Can you work these out from the model? Positions are in its coordinate system, mm. A direction names the side the tool comes from. Coordinates: 2 decimals unless noted, no trailing zeros. Order: outer loops, then holes, each group sorted by start corner. A loop starts at its lowest first (then second) coordinate and runs counter-clockwise, first axis right, second up. Notation, with made-up numbers: (73, 20.25) -> (81, 20.25) arc R28 ccw to (81, 39.25) -> close; hole circle Ø4 at (51.5, 17). An arc over 180 degrees is marked (long way). Answer as a JSON object with one key per item and string values. Group by question number.
(1) I want a section at C-C, the plane x = -25. List the corners of the cut face in (y, z) for me.
(2) For pin 1 (1.5 mm diameter, centred on x = -16.5, z = 11, fed in from -Y); pin 2 (1.3 mm diameter, centred on x = -11.5, z = -2.5, fed in from -Y); pin 3 (12 mm diameter, centred on y = -8.5, z = -16.5, fed in from +X); pin 4 (1.5 mm diameter, centred on y = -1.5, z = -11.5, fed in from -X), each with a flat end and sliding along its axis, tell me the tip position at first contact or that it passes through.
(3) I want a section at A-A, the plane y = 5.5. List the corners of the cut face in (x, z) for me, plus the area to 3 significant figures.
(4) Which directions (+Z, -Z, +X, -X, +Y, -Y) give clear straight access to the entire face, cutting with the end or side of a thin tool? Please do faces 4 (the flat face through (11, -5, 0)), 5 (the flat face through (-11, -5, 0)), 6 (the flat face through (0, -5, -11)), 7 (the flat face through (0, -5, 11)).
(5) I want a section at D-D, the plane y = -0.75. List the corners of the cut face in (x, z) for me, plus the area to 3 significant figures.
(6) I need wall thicknesses on line 1 (X direction, y = -9, z = 13.5); line 2 (Z direction, x = 23, y = -11.25); line 3 (Y direction, x = 12, z = 3). Which ranges of each line are inside material? Lowest first, please.
(7) If we mould it in two halves opening along Z, with no side actions, what happens to faces 1 (the cylindrical face through (21.166, -8.944, 21.26)), 2 (the cylindrical face through (8.64, 4.06, -9.08)), 3 (the flat face through (-15, -5, -15))? For each: pulls with the +Z half, pulls with the -Z half, needs draft (parallel to the pull), parting line crosses it, or undercut.
(8) I want a section at B-B, the plane z = -15. State how many separate pieces and enclosed holes the cut face has, plus the area to 3 significant figures.
Autodesk Inventor part; units mm, degrees
ref_plane "YZ Plane" through (0, 0, 0) normal (1, 0, 0) x (0, 1, 0)
ref_plane "XZ Plane" through (0, 0, 0) normal (0, 1, 0) x (-1, 0, 0)
ref_plane "XY Plane" through (0, 0, 0) normal (0, 0, 1) x (1, 0, 0)
sketch "スケッチ1" plane through (0, 0, 0) normal (0, 1, 0) x (-1, 0, 0)
  circle A0 centre (0, 0) radius 25
  circle A1 centre (0, 0) radius 30
  dimension "d0" = 50
  dimension "d1" = 60
extrude "押し出し1" add sketch "スケッチ1" along normal blind 8 contours A0 | A1
sketch "スケッチ2" plane through (0, 8, 0) normal (0, 1, 0) x (1, 0, 0)
  circle A0 centre (0, 0) radius 30
  line L0 (0, -30) -> (-30, 0)
  line L1 (-30, 0) -> (0, 30)
  line L2 (0, 30) -> (30, 0)
  line L3 (0, -30) -> (30, 0)
  circle A1 centre (0, 0) radius 30
  circle A2 centre (0, 0) radius 25
  circle A3 centre (-23, 23) radius 20
  circle A4 centre (-23, -23) radius 20
  circle A5 centre (23, -23) radius 20
  circle A6 centre (23, 23) radius 20
  point P0 (-4.1593, 29.7103)
  point P1 (-29.7103, 4.1593)
  dimension "d5" = 50
  dimension "d8" = 23
  dimension "d9" = 23
  dimension "d13" = 360
  dimension "d29" = 40
extrude "押し出し2" cut sketch "スケッチ2" against normal blind 10 contours A6 L2 A2 A0 | A0 A6 | A5 A0 | A0 A5 L3 A2 | A6 A2 L2 | L3 A2 A5 | A2 A6 L2 | L2 A2 | A2 L3 | L3 A2 A5 | L2 A2 A6 | A5 A2 L3 | A3 L1 A2 A0 | A0 A3 | A3 A2 L1 | A4 A0 | A0 A4 L0 A2 | L0 A2 A4 | A3 A2 L1 | A2 L0 A4 | L1 A2 | A2 L0 | L1 A2 A3 | A4 A2 L0
sketch "スケッチ3" plane through (0, 8, 0) normal (0, 1, 0) x (1, 0, 0)
  line L0 (0, -0.0001) -> (0, -29.9755)
  circle A0 centre (-0.0169, 0.0244) radius 30
  line L1 (0, -0.0001) -> (32.5269, -32.527)
  line L2 (32.5269, -32.527) -> (0, -32.527)
  line L3 (21.1924, -21.1926) -> (0, -21.1926)
  ellipse E0 centre (0, -32.527) end of major axis (20.2314, -32.527) minor radius 22.6164
  ellipse E1 centre (32.5345, 0.0414) end of major axis (32.5345, 20.2728) minor radius 22.6164
  ellipse E2 centre (-0.0339, 32.5759) end of major axis (-20.2653, 32.5759) minor radius 22.6164
  ellipse E3 centre (-32.5684, 0.0075) end of major axis (-32.5684, -20.2239) minor radius 22.6164
  point P0 (0, 0)
  point P1 (-4.1509, 30.0937)
  point P2 (-30.9256, 3.319)
  dimension "d50" = 21.1925
  dimension "d51" = 360
sketch "スケッチ4" plane through (0, 0, 0) normal (0, -1, 0) x (1, 0, 0)
  circle A0 centre (0, 0) radius 12.5
  dimension "d15" = 25
extrude "押し出し3" add sketch "スケッチ4" along normal blind 5
sketch "スケッチ5" plane through (0, -5, 0) normal (0, -1, 0) x (1, 0, 0)
  circle A0 centre (0, 0) radius 30
  dimension "d18" = 60
extrude "押し出し4" add sketch "スケッチ5" along normal blind 8
sketch "スケッチ6" plane through (0, -13, 0) normal (0, -1, 0) x (1, 0, 0)
  line L0 (0.0169, -0.0245) -> (0.0169, -30)
  circle A0 centre (0, 0) radius 30
  line L1 (0.0169, -0.0245) -> (32.5438, -32.5514)
  line L2 (32.5438, -32.5514) -> (0.0169, -32.5514)
  line L3 (21.2094, -21.217) -> (0.0169, -21.217)
  ellipse E0 centre (0.0169, -32.5514) end of major axis (20.2483, -32.5514) minor radius 22.6164
  ellipse E1 centre (32.5514, 0.0169) end of major axis (32.5514, 20.2483) minor radius 22.6164
  ellipse E2 centre (-0.0169, 32.5514) end of major axis (-20.2483, 32.5514) minor radius 22.6164
  ellipse E3 centre (-32.5514, -0.0169) end of major axis (-32.5514, -20.2483) minor radius 22.6164
  point P0 (-3.3011, 29.5474)
  point P1 (-30.0758, 2.7727)
  dimension "d43" = 21.1925
  dimension "d46" = 360
extrude "押し出し5" cut sketch "スケッチ6" against normal blind 8 contours E0 L3 L0 | L0 A0 E0 | L3 E0 A0 L0 | A0 E0 | E1 A0 | A0 E1 | E3 A0 | A0 E3 | E2 A0 | A0 E2
Computed values:
{
 "1": {"outline": "(0, -3.1) -> (8, -3.1) -> (8, 3.1) -> (0, 3.1) -> close"},
 "2": {"pin 1": "passes through", "pin 2": "stops at y = -5", "pin 3": "stops at x = 23.58", "pin 4": "stops at x = -6.38"},
 "3": {"outline": "(-29.71, -4.16) arc R20 cw to (-4.16, -29.71) arc R30 ccw to (4.16, -29.71) arc R20 cw to (29.71, -4.16) arc R30 ccw to (29.71, 4.16) arc R20 cw to (4.16, 29.71) arc R30 ccw to (-4.16, 29.71) arc R20 cw to (-29.71, 4.16) arc R30 ccw to start", "area": "1,050 mm2"},
 "4": {"face 4": "+X, -Y", "face 5": "-X, -Y", "face 6": "-Z, -Y", "face 7": "+Z, -Y"},
 "5": {"outline": "circle Ø25 at (0, 0)", "area": "491 mm2"},
 "6": {"line 1": "x = -15.72 to -10.92, 10.89 to 15.69", "line 2": "z = -19.26 to -18.32, 18.36 to 19.26", "line 3": "y = -5 to 8"},
 "7": {"face 1": "pulls with the +Z half", "face 2": "undercut", "face 3": "needs draft"},
 "8": {"separate pieces": "3", "enclosed holes": "0", "area": "149 mm2"}
}
